Check sheet for the modelled part. Datum: model origin and axes. Units: mm. Face numbers are marked on the shaded views. A direction names the side the tool comes from. Coordinates: 2 decimals unless noted, no trailing zeros. Order: outer loops, then holes, each group sorted by start corner. A loop starts at its lowest first (then second) coordinate and runs counter-clockwise, first axis right, second up. Notation, with made-up numbers: (-0.5, 43) -> (54.5, 43) arc R17 cw to (54.5, 76) -> close; hole circle Ø1 at (-35, 86.5). An arc over 180 degrees is marked (long way). Put each result on its own line as item: value. Start each with the question number.
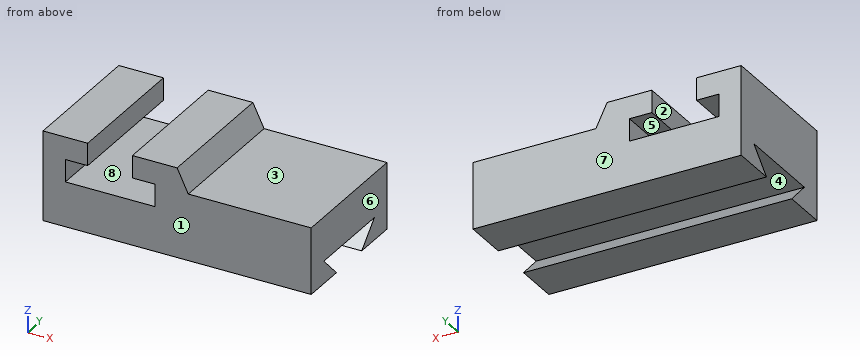
```python
from build123d import *

# Parameters (mm, degrees)
F0_W     = 152.4
F0_H     = 50.8
F1_DEPTH = 76.2
F3_DEPTH = 76.2
F5_DEPTH = 152.4


with BuildPart() as f1:
    # F0 (on Front) → F1 (new body)
    with BuildSketch(Plane.XZ):
        with Locations((76.2, 25.4)):
            Rectangle(F0_W, F0_H)
    extrude(amount=-F1_DEPTH)

    # F2 (on face) → F3 (cut)
    with BuildSketch(Plane.XZ):
        Polygon((50.8, 50.8), (25.4, 50.8), (25.4, 38.1), (12.700001, 38.1), (12.700001, 25.4), (63.500001, 25.4), (63.500001, 38.1), (50.8, 38.1), align=None)
        Polygon((82.55, 37.719), (152.4, 37.719), (152.4, 50.8), (76.2, 50.8), align=None)
    extrude(amount=-F3_DEPTH, mode=Mode.SUBTRACT)

    # F4 (on face) → F5 (cut)
    with BuildSketch(Plane.YZ.offset(152.4)):
        Polygon((12.7, 12.7), (25.4, 0), (50.8, 0), (63.5, 12.7), align=None)
    extrude(amount=-F5_DEPTH, mode=Mode.SUBTRACT)


solid = f1.part
```
1) Sectioned sample at A-A (y = 17.5). Record the boundary of the cut face in (x, z), plus the area to 3 significant figures.
2) Sectioned sample at C-C (z = 11). Record the boundary of the cut face in (x, y), plus the area to 3 significant figures.
3) Mould release check, pull along X, two halves, no side actions. Record for the marked faces 6, 7 and 8: +X half, -X half, draft (parallel to the pull), parting line (faces both ways), or undercut.
4) Gauge pin test, flat ends, axial feed: pin 1 (14 mm diameter, centred on x = 16, y = 35, fed in from -Z); pin 2 (10 mm diameter, centred on y = 22.5, z = 46, fed in from +X). Record the tip position at first contact, or that the pin passes through.
5) Sectioned sample at D-D (x = 122.5). Record the boundary of the cut face in (y, z), plus the area to 3 significant figures.
6) Sectioned sample at B-B (x = 56). Record the boundary of the cut face in (y, z).
7) Scan lines: line 1 along Z through (x, y) = (61, 73.5); line 2 along Z through (x, y) = (16, 51); line 3 along X through (y, z) = (71, 36.5). Record each from-to range of solid material in increasing order. Write a range as [from, to].
8) Access from +Z, -Z, +X, -X, +Y, -Y to the whole of each face (thin tool, end or side, straight path). Record for the marked faces 1, 2, 3, 4 and 5.
Entries:
1. outline: (0, 0) -> (152.4, 0) -> (152.4, 7.9) -> (0, 7.9) -> close; (0, 12.7) -> (152.4, 12.7) -> (152.4, 37.72) -> (82.55, 37.72) -> (76.2, 50.8) -> (50.8, 50.8) -> (50.8, 38.1) -> (63.5, 38.1) -> (63.5, 25.4) -> (12.7, 25.4) -> (12.7, 38.1) -> (25.4, 38.1) -> (25.4, 50.8) -> (0, 50.8) -> close
1. area: 5,090 mm2
2. outline: (0, 0) -> (152.4, 0) -> (152.4, 14.4) -> (0, 14.4) -> close; (0, 61.8) -> (152.4, 61.8) -> (152.4, 76.2) -> (0, 76.2) -> close
2. area: 4,390 mm2
3. face 6: +X half
3. face 7: draft
3. face 8: undercut
4. pin 1: stops at z = 12.7
4. pin 2: stops at x = 80.96
5. outline: (0, 0) -> (25.4, 0) -> (12.7, 12.7) -> (63.5, 12.7) -> (50.8, 0) -> (76.2, 0) -> (76.2, 37.72) -> (0, 37.72) -> close
5. area: 2,390 mm2
6. outline: (0, 0) -> (25.4, 0) -> (12.7, 12.7) -> (63.5, 12.7) -> (50.8, 0) -> (76.2, 0) -> (76.2, 25.4) -> (0, 25.4) -> close; (0, 38.1) -> (76.2, 38.1) -> (76.2, 50.8) -> (0, 50.8) -> close
7. line 1: z = [0, 25.4], [38.1, 50.8]
7. line 2: z = [0, 0.2], [12.7, 25.4], [38.1, 50.8]
7. line 3: x = [0, 12.7], [63.5, 152.4]
8. face 1: +Z, -Z, +X, -X, -Y
8. face 2: +Z, +Y, -Y
8. face 3: +Z, +X, +Y, -Y
8. face 4: +X, -X
8. face 5: +Y, -Y
